For this review, take the finished solid that the model builds, in its own axes (mm). Coordinates: 2 decimals unless noted, no trailing zeros. One line per item, written item: value. Start each with the question number.
1) For probe 1 along X at (y, z) = (16.5, 1.8); probe 2 along Y at (x, z) = (-29, 0.75); probe 3 along X at (y, z) = (-27.5, 0.2), list the stretches that pass through material, from the lowest coordinate up. Write a range as from..to.
2) Mouldability with a two-part tool opening along Y and no side actions: class faces 1 (the cylindrical face through (-32.885, -16.563, 0.967)), 2 (the flat face through (-1, 0, 3.175)), 3 (the flat face through (0, 33.084, 2)), 4 (the cylindrical face through (32.74, -16.31, 0.97)) as released by +Y, released by -Y, zero draft, split by the parting line, or undercut.
3) For pin 1 Ø3.5 at (x, y) = (-33.782, 15.875) entering from +Z; pin 2 Ø2 at (x, y) = (-15.875, -30.607) entering from -Z; pin 3 Ø12 at (x, y) = (13, 2) entering from -Z; pin 4 Ø3 at (x, y) = (15.875, -30.607) entering from +Z, all flat-tipped, find the tip position at first contact; note any pin that passes through.
4) Add section A-A (z = 1.45). State how many separate pieces and enclosed holes the cut face has, and give its area (3 significant figures).
from build123d import *

# Parameters (mm, degrees)
BOSS_EXTRUDE1_DEPTH                            = 3.175
CSK_FOR_2_FLAT_HEAD_MACHINE_SCREW1_D           = 2.2606
CSK_FOR_2_FLAT_HEAD_MACHINE_SCREW1_CSINK_D     = 4.3688
CSK_FOR_2_FLAT_HEAD_MACHINE_SCREW1_CSINK_ANGLE = 82


with BuildPart() as part:
    # Sketch1 → Boss-Extrude1 (new body)
    with BuildSketch(Plane.XY):
        with BuildLine():
            Line((-36.2585, 25.4), (-36.2585, -25.4))
            ThreePointArc((-36.2585, -25.4), (-34.008054953, -30.833054953), (-28.575, -33.0835))
            Line((-28.575, -33.0835), (28.575, -33.0835))
            ThreePointArc((28.575, -33.0835), (34.008054953, -30.833054953), (36.2585, -25.4))
            Line((36.2585, -25.4), (36.2585, 25.4))
            ThreePointArc((36.2585, 25.4), (34.008054953, 30.833054953), (28.575, 33.0835))
            Line((28.575, 33.0835), (-28.575, 33.0835))
            ThreePointArc((-28.575, 33.0835), (-34.008054953, 30.833054953), (-36.2585, 25.4))
        make_face()
    extrude(amount=BOSS_EXTRUDE1_DEPTH)

    # CSK for #2 Flat Head Machine Screw1 (through all)
    with Locations(Plane(origin=(13.435602358, 90.246811513, 3.175), x_dir=(1, 0, 0), z_dir=(0, 0, 1))):
        with Locations((-29.310602358, -59.639811513), (-47.217602358, -74.371811513), (-47.217602358, -106.121811513), (-29.310602358, -120.853811513), (2.439397642, -120.853811513), (20.346397642, -106.121811513), (20.346397642, -74.371811513), (2.439397642, -59.639811513)):
            CounterSinkHole(CSK_FOR_2_FLAT_HEAD_MACHINE_SCREW1_D / 2, CSK_FOR_2_FLAT_HEAD_MACHINE_SCREW1_CSINK_D / 2, counter_sink_angle=CSK_FOR_2_FLAT_HEAD_MACHINE_SCREW1_CSINK_ANGLE)


solid = part.part
Numbers:
1. probe 1: -36.26..-34.72, -32.84..32.84, 34.72..36.26
1. probe 2: -33.07..33.07
1. probe 3: -35.97..35.97
2. face 1: undercut
2. face 2: zero draft
2. face 3: released by +Y
2. face 4: undercut
3. pin 1: z = 2.68
3. pin 2: through
3. pin 3: z = 0
3. pin 4: z = 2.39
4. separate pieces: 1
4. enclosed holes: 8
4. area: 4,720 mm²
